from build123d import *

# Parameters (mm, degrees)
CROQUIS1_W              = 30
CROQUIS1_H              = 30
SALIENTE_EXTRUIR1_DEPTH = 30
CROQUIS2_R              = 12.5
CORTAR_EXTRUIR1_DEPTH   = 30
CROQUIS4_W              = 30
CROQUIS4_H              = 30
SALIENTE_EXTRUIR5_DEPTH = 17.5
CROQUIS6_W              = 30
CROQUIS6_H              = 25
CORTAR_EXTRUIR3_DEPTH   = 37.5
CROQUIS7_R              = 4.5
CORTAR_EXTRUIR5_DEPTH   = 37.5
CROQUIS8_R              = 2
SALIENTE_EXTRUIR6_DEPTH = 2.5
CROQUIS9_W              = 26.5
CROQUIS9_H              = 8
CROQUIS9_R              = 2
SALIENTE_EXTRUIR7_DEPTH = 2.5
REDONDEO1_R             = 2.5


with BuildPart() as part:
    # Croquis1 → Saliente-Extruir1 (new body)
    with BuildSketch(Plane(origin=(0, 0, 0), x_dir=(1, 0, 0), z_dir=(0, 1, 0))):
        Rectangle(CROQUIS1_W, CROQUIS1_H)
    extrude(amount=SALIENTE_EXTRUIR1_DEPTH)

    # Croquis2 → Cortar-Extruir1 (cut)
    with BuildSketch(Plane(origin=(0, 30, 0), x_dir=(1, 0, 0), z_dir=(0, 1, 0))):
        Circle(CROQUIS2_R)
    extrude(amount=-CORTAR_EXTRUIR1_DEPTH, mode=Mode.SUBTRACT)

    # Croquis4 → Saliente-Extruir5 (add)
    with BuildSketch(Plane.ZY.offset(15)):
        with Locations((0, 15)):
            Rectangle(CROQUIS4_W, CROQUIS4_H)
    extrude(amount=SALIENTE_EXTRUIR5_DEPTH)

    # Croquis6 → Cortar-Extruir3 (cut)
    with BuildSketch(Plane(origin=(0, 30, 0), x_dir=(1, 0, 0), z_dir=(0, 1, 0))):
        with Locations((-15, 0)):
            Rectangle(CROQUIS6_W, CROQUIS6_H)
    extrude(amount=-CORTAR_EXTRUIR3_DEPTH, mode=Mode.SUBTRACT)

    # Croquis7 → Cortar-Extruir5 (cut)
    with BuildSketch(Plane(origin=(0, 0, -15), x_dir=(-1, 0, 0), z_dir=(0, 0, -1))):
        with Locations((18, 15)):
            Circle(CROQUIS7_R)
    extrude(amount=-CORTAR_EXTRUIR5_DEPTH, mode=Mode.SUBTRACT)

    # Croquis8 → Saliente-Extruir6 (add)
    with BuildSketch(Plane.XY.offset(15)):
        with BuildLine():
            Line((-36.03122292, 25.717514421), (-32.5, 25.717514421))
            Line((-32.5, 25.717514421), (-32.5, 17.717514421))
            Line((-32.5, 17.717514421), (-36.03122292, 17.717514421))
            ThreePointArc((-36.03122292, 17.717514421), (-40.03122292, 21.717514421), (-36.03122292, 25.717514421))
        make_face()
        with Locations((-36.03122292, 21.717514421)):
            Circle(CROQUIS8_R, mode=Mode.SUBTRACT)
        with BuildLine():
            Line((-15.282485579, -3.03122292), (-15.282485579, 0))
            Line((-15.282485579, 0), (-7.282485579, 0))
            Line((-7.282485579, 0), (-7.282485579, -3.03122292))
            ThreePointArc((-7.282485579, -3.03122292), (-11.282485579, -7.03122292), (-15.282485579, -3.03122292))
        make_face()
        with Locations((-11.282485579, -3.03122292)):
            Circle(CROQUIS8_R, mode=Mode.SUBTRACT)
    extrude(amount=-SALIENTE_EXTRUIR6_DEPTH)

    # Croquis9 → Saliente-Extruir7 (add)
    with BuildSketch(Plane(origin=(0, 30, 0), x_dir=(1, 0, 0), z_dir=(0, 1, 0))):
        with Locations((-8.75, 19)):
            Rectangle(CROQUIS9_W, CROQUIS9_H)
        with Locations((0, 18.5)):
            Circle(CROQUIS9_R, mode=Mode.SUBTRACT)
        with Locations((-17.5, 18.5)):
            Circle(CROQUIS9_R, mode=Mode.SUBTRACT)
        with Locations((-8.75, -19)):
            Rectangle(CROQUIS9_W, CROQUIS9_H)
        with Locations((0, -18.5)):
            Circle(CROQUIS9_R, mode=Mode.SUBTRACT)
        with Locations((-17.5, -18.5)):
            Circle(CROQUIS9_R, mode=Mode.SUBTRACT)
    extrude(amount=-SALIENTE_EXTRUIR7_DEPTH)

    # Redondeo1
    redondeo1_edges = [part.edges().sort_by_distance(p)[0] for p in [
        (-22, 28.75, 23),
        (-22, 28.75, 15),
        (4.5, 28.75, 15),
        (4.5, 28.75, 23),
        (-22, 28.75, -15),
        (-22, 28.75, -23),
        (4.5, 28.75, -23),
        (4.5, 28.75, -15),
    ]]
    fillet(redondeo1_edges, radius=REDONDEO1_R)


solid = part.part
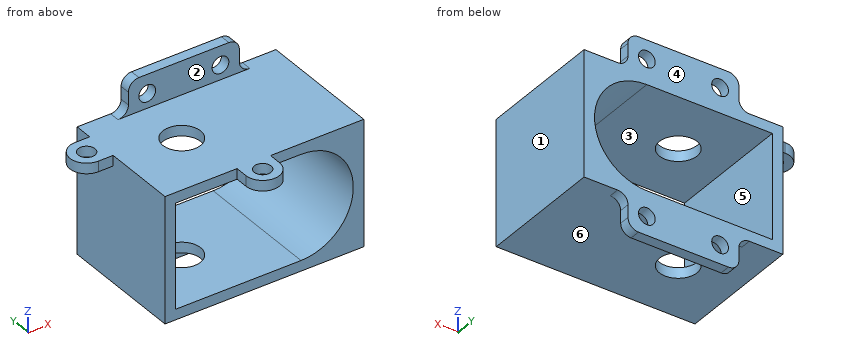
Work out the finished part from the listing and answer in its coordinate system (mm). Face numbers are marked on the shaded views. A direction names the side the tool comes from. Give positions to 0.01 mm unless a question says otherwise; leave off trailing zeros. Write each loop counter-clockwise with the first axis right and the second up, starting at its lowest first coordinate (ties: lowest second). Pieces come first, ordered by that corner, then holes. Notation, with made-up numbers: M 56,-33 L 107,-33 A12 cw 107,-24 Z; hole C 26.25,55.5 d4. An arc over 180 degrees is marked long. Answer as CSV lines item,"result".
Q1. Given P1, Ø8.5, axis at x = -38, y = 21, coming from the -Z side; P2, Ø1.5, axis at x = 3.5, y = 4.5, coming from the -Z side; P3, Ø2, axis at y = 29, z = 19.5, coming from the +X side, each flat-ended and moving along its own axis, determine where each tip first touches the part or whether it passes through.
A:
P1,"stops at z = 12.5"
P2,"stops at z = -15"
P3,"stops at x = 4.5"
Q2. A cutting plane is placed at D-D on x = -17.5. Write down the section's boundary in (y, z), plus the area to 3 significant figures.
A:
outline,"M 0,-15 L 10.53,-15 L 10.53,-12.5 L 0,-12.5 Z; M 0,12.5 L 10.53,12.5 L 10.53,15 L 0,15 Z; M 19.47,-15 L 27.5,-15 L 27.5,-16.5 L 30,-16.5 L 30,-12.5 L 19.47,-12.5 Z; M 19.47,12.5 L 30,12.5 L 30,16.5 L 27.5,16.5 L 27.5,15 L 19.47,15 Z; M 27.5,-23 L 30,-23 L 30,-20.5 L 27.5,-20.5 Z; M 27.5,20.5 L 30,20.5 L 30,23 L 27.5,23 Z"
area,"125 mm²"
Q3. The mould has two halves that part along Z. Classify the marked faces 4, 5 and 6: +Z half, -Z half, draft (parallel to the pull), parting line (faces both ways), or undercut.
A:
face 4,"draft"
face 5,"undercut"
face 6,"-Z half"
Q4. A tool of negligible diameter and unlimited length cuts with its end or side. For the marked faces 1, 2 and 3, from which of +Z, -Z, +X, -X, +Y, -Y can it reach the whole face along a straight path? Write none if from no direction.
A:
face 1,"+Z, -Z, +X, +Y, -Y"
face 2,"+Z, +X, -X, -Y"
face 3,"+Y, -Y"
Q5. A cutting plane is placed at B-B on y = 15. Write down the section's boundary in (x, z), plus the area to 3 significant figures.
A:
outline,"M -32.5,-15 L -22.5,-15 L -22.5,-12.5 L -30,-12.5 L -30,12.5 L -22.5,12.5 L -22.5,15 L -32.5,15 Z; M -13.5,-15 L 15,-15 L 15,15 L -13.5,15 L -13.5,12.5 L 0,12.5 A12.5 cw 0,-12.5 L -13.5,-12.5 Z"
area,"385 mm²"
Q6. A cutting plane is placed at C-C on z = 0. Write down the section's boundary in (x, y), plus the area to 3 significant figures.
A:
outline,"M -32.5,0 L -30,0 L -30,30 L -32.5,30 Z; M 12.5,0 L 15,0 L 15,30 L 12.5,30 Z"
area,"150 mm²"
Q7. A cutting plane is placed at A-A on z = -18.5. Write down the section's boundary in (x, y).
A:
outline,"M -22,27.5 L -19.5,27.5 L -19.5,30 L -22,30 Z; M -15.5,27.5 L -2,27.5 L -2,30 L -15.5,30 Z; M 2,27.5 L 4.5,27.5 L 4.5,30 L 2,30 Z"
Q8. Find the intervals of material crossed by probe 1 along X at (y, z) = (28.2, 18.5); probe 2 along Z at (x, y) = (0, 28.1); probe 3 along Z at (x, y) = (-5.5, 3), in increasing order. Write a range as [from, to].
A:
probe 1,"x = [-22, -19.5], [-15.5, -2], [2, 4.5]"
probe 2,"z = [-23, -20.5], [-16.5, -12.5], [12.5, 16.5], [20.5, 23]"
probe 3,"z = [-15, -12.5], [12.5, 15]"
